Could you check a few things on this model? Use its own coordinates, in mm. A direction names the side the tool comes from. Coordinates: 2 decimals unless noted, no trailing zeros. Write each loop counter-clockwise with the first axis right and the second up, starting at its lowest first coordinate (ties: lowest second). Pieces come first, ordered by that corner, then holes.
```python
from build123d import *

# Parameters (mm, degrees)
ESBO_O1_W                = 20
ESBO_O1_H                = 22
RESSALTO_EXTRUS_O1_DEPTH = 1.5
ESBO_O2_R                = 8
RESSALTO_EXTRUS_O2_DEPTH = 14
FILETE1_R                = 2
ESBO_O3_R                = 2.5
RESSALTO_EXTRUS_O3_DEPTH = 21
ESBO_O4_W                = 8
ESBO_O4_H                = 8
RESSALTO_EXTRUS_O4_DEPTH = 10


with BuildPart() as part:
    # Esboço1 → Ressalto-extrusão1 (new body)
    with BuildSketch(Plane(origin=(0, 0, 0), x_dir=(1, 0, 0), z_dir=(0, 1, 0))):
        with Locations((-0.363033398, -2.207136461)):
            Rectangle(ESBO_O1_W, ESBO_O1_H)
    extrude(amount=RESSALTO_EXTRUS_O1_DEPTH)

    # Esboço2 → Ressalto-extrusão2 (add)
    with BuildSketch(Plane(origin=(0, 1.5, 0), x_dir=(1, 0, 0), z_dir=(0, 1, 0))):
        with Locations((0, -1.584818961)):
            Circle(ESBO_O2_R)
    extrude(amount=RESSALTO_EXTRUS_O2_DEPTH)

    # Filete1
    filete1_edges = [part.edges().sort_by_distance(p)[0] for p in [
        (-8, 15.5, 1.584818961),
    ]]
    fillet(filete1_edges, radius=FILETE1_R)

    # Esboço3 → Ressalto-extrusão3 (add)
    with BuildSketch(Plane(origin=(0, 0, 0), x_dir=(-1, 0, 0), z_dir=(0, -1, 0))):
        with Locations((7.446149428, -10.420452969)):
            Circle(ESBO_O3_R)
        with Locations((-6.479235285, 5.224259997)):
            Circle(ESBO_O3_R)
    extrude(amount=RESSALTO_EXTRUS_O3_DEPTH)

    # Esboço4 → Ressalto-extrusão4 (add)
    with BuildSketch(Plane(origin=(0, 0, 0), x_dir=(-1, 0, 0), z_dir=(0, -1, 0))):
        with Locations((4.363033398, 0.792863539)):
            Rectangle(ESBO_O4_W, ESBO_O4_H)
    extrude(amount=RESSALTO_EXTRUS_O4_DEPTH)


solid = part.part
```
Item 1: I want a section at B-B, the plane y = -19. List the corners of the cut face in (x, z) for me, then the cut area to 3 significant figures.
Item 2: I want a section at C-C, the plane y = 2. List the corners of the cut face in (x, z) for me.
Item 3: Will these pins go through, and if not, where does the flat tip stop? pin 1 Ø6.5 at (x, y) = (-3.5, -5.5) entering from -Z; pin 2 Ø3 at (x, y) = (4, -8) entering from -Z; pin 3 Ø2 at (y, z) = (8.5, 10) entering from +X; pin 4 Ø10 at (y, z) = (-3, 7) entering from +X.
Item 4: If we mould it in two halves opening along Z, with no side actions, what happens to faces 5 (the cylindrical face through (-8.79, -10.35, 8.31)), 6 (the flat face through (-7, -21, 10)), 7 (the flat face through (-4, -5, -4.793))? For each: released by +Z, released by -Z, zero draft, split by the parting line, or undercut.
Item 5: Which directions (+Z, -Z, +X, -X, +Y, -Y) give clear straight access to the entire face, cutting with the end or side of a thin tool? Please do faces 1 (the cylindrical face through (7.021, -10.353, -2.784)), 2 (the flat face through (-4, -5, 3.207)), 3 (the flat face through (-0.363, -5, -1)), 4 (the flat face through (-4, -10, -1)).
Item 6: If I drill on line 1 along Y through (x, z) = (-9, -7.5); line 2 along Z through (x, y) = (-3, -7.5); line 3 along Y through (x, z) = (-4.25, 3.25), over which ranges is the centre line in solid material (lowest first)?
Item 7: I want a section at A-A, the plane y = -3. List the corners of the cut face in (x, z) for me.
Taken from the geometry:
1. outline: circle Ø5 at (-7.45, 10.42); circle Ø5 at (6.48, -5.22)
1. area: 39.3 mm2
2. outline: circle Ø16 at (0, 1.58)
3. pin 1: stops at z = -4.79
3. pin 2: stops at z = -7.52
3. pin 3: stops at x = 3
3. pin 4: stops at x = 9.64
4. face 5: undercut
4. face 6: zero draft
4. face 7: released by -Z
5. face 1: -Y
5. face 2: +X, -X, -Y
5. face 3: +Z, -Z, -Y
5. face 4: -Z, -X, -Y
6. line 1: y = 0 to 1.5
6. line 2: z = -4.79 to 3.21
6. line 3: y = 0 to 15.5
7. outline: circle Ø5 at (-7.45, 10.42); (-8.36, -4.79) - (-0.36, -4.79) - (-0.36, 3.21) - (-8.36, 3.21) - close; circle Ø5 at (6.48, -5.22)
